The model under review builds one solid part; all positions refer to its coordinate system, in mm. A direction names the side the tool comes from. Coordinates: 2 decimals unless noted, no trailing zeros. Loops run counter-clockwise (first coordinate to the right, second up) from the corner with the lowest first, then second, coordinate; pieces in that order, holes last. Notation, with made-up numbers: M 75.25,-36 L 125.25,-36 A17 ccw 125.25,-17 Z; hole C -22.5,68.25 d10. An arc over 180 degrees is marked long. Use one line per item in the form item = value.
```python
from build123d import *

# Parameters (mm, degrees)
F1_DEPTH = 609.6
F2_R     = 5.08


with BuildPart() as f1:
    # F0 (on Front) → F1 (new body)
    with BuildSketch(Plane.XZ):
        Polygon((-76.2, -46.21704), (-76.2, -57.094753), (76.2, -57.094753), (76.2, -46.21704), (26.83735, -33.72637), (21.163462, -31.835258), (18.708812, -29.612178), (16.218112, -26.55388), (14.689744, -22.895062), (13.485576, -19.143616), (13.305501, -16.85449), (10.935693, -2.660843), (9.173225, 23.941404), (9.095304, 51.274587), (9.465817, 61.371074), (10.203332, 68.52603), (11.415046, 73.405639), (12.987001, 77.66302), (14.984693, 80.446691), (18.095852, 83.001115), (20.683027, 84.147327), (25.922873, 85.98128), (30.180251, 87.1275), (33.094916, 87.749728), (34.175634, 88.306465), (35.387348, 89.616426), (36.173157, 90.991981), (36.40228, 91.97448), (36.598587, 93.513711), (36.598872, 93.52041), (36.827176, 98.88458), (36.669851, 103.667696), (36.407496, 106.64783), (36.177806, 110.315693), (35.555092, 114.278253), (34.24468, 117.978737), (33.327476, 119.878062), (31.132972, 122.464971), (28.218115, 124.036569), (24.026078, 125.34602), (19.539378, 126.000454), (15.433662, 126.392808), (7.999516, 126.762047), (0, 126.762047), (-7.999516, 126.762047), (-15.433662, 126.392808), (-19.539378, 126.000454), (-24.026078, 125.34602), (-28.218115, 124.036569), (-31.132972, 122.464971), (-33.327476, 119.878062), (-34.24468, 117.978737), (-35.555092, 114.278253), (-36.177806, 110.315693), (-36.407496, 106.64783), (-36.669851, 103.667696), (-36.827176, 98.88458), (-36.598872, 93.52041), (-36.598587, 93.513711), (-36.40228, 91.97448), (-36.173157, 90.991981), (-35.387348, 89.616426), (-34.175634, 88.306465), (-33.094916, 87.749728), (-30.180251, 87.1275), (-25.922873, 85.98128), (-20.683027, 84.147327), (-18.095852, 83.001115), (-14.984693, 80.446691), (-12.987001, 77.66302), (-11.415046, 73.405639), (-10.203332, 68.52603), (-9.465817, 61.371074), (-9.095304, 51.274587), (-9.173225, 23.941404), (-10.935693, -2.660843), (-13.305501, -16.85449), (-13.485576, -19.143616), (-14.689744, -22.895062), (-16.218112, -26.55388), (-18.708812, -29.612178), (-21.163462, -31.835258), (-26.83735, -33.72637), align=None)
    extrude(amount=F1_DEPTH)

    # F2
    f2_edges = [f1.edges().sort_by_distance(p)[0] for p in [
        (76.2, -304.8, -46.21704),
        (-76.2, -304.8, -46.21704),
    ]]
    fillet(f2_edges, radius=F2_R)


solid = f1.part
```
1. Wall thickness on line 1 along X through (y, z) = (-460.5, 6.5); line 2 along Z through (x, y) = (-32, -50); line 3 along X through (y, z) = (-153, 96): over which ranges is each line inside the solid? List them lowest first. Write a range as from..to.
Response values:
line_1 = -10.33..10.33
line_2 = -57.09..-35.03, 87.52..121.44
line_3 = -36.7..36.7
2. Insertion check: P1, Ø4, axis at y = -84.5, z = 80.5, coming from the +X side; P2, Ø5, axis at y = -372.5, z = 104, coming from the -X side; P3, Ø12, axis at y = -184.5, z = 86.5, coming from the +X side. Each pin has a flat end and moves straight along its axis. Give the tip position at first contact, or say it passes through.
Response values:
P1 = 17.49
P2 = -36.74
P3 = 36.47
3. The part is to be moulded in two halves that separate along Z. For faces 4 (the face through (0, 0, 28)), 5 (the face through (-12.104, -300.533, -9.658)), 6 (the face through (12.137, -300.533, -9.857)), 7 (the face through (-1, -301, -57.095)), say which applies: pulls with the +Z half, pulls with the -Z half, needs draft (parallel to the pull), parting line crosses it, or undercut.
Response values:
face_4 = needs draft
face_5 = undercut
face_6 = undercut
face_7 = pulls with the -Z half
4. Add section B-B (x = 56). State the section outline as (y, z) points, then the cut area to 3 significant figures.
Response values:
outline = M -609.6,-57.09 L 0,-57.09 L 0,-41.11 L -609.6,-41.11 Z
area = 9,750 mm^2
5. Machinability: for faces 1 (the face through (-49.283, -300.533, -39.406)), 2 (the face through (49.92, -300.533, -39.567)), 3 (the face through (0, -301, 126.762)), which of the approach directions +Z, -Z, +X, -X, +Y, -Y give a long, thin tool a straight path to every point of the face, cutting with its end or side? Answer none if there is none.
Response values:
face_1 = -X, +Y, -Y
face_2 = +X, +Y, -Y
face_3 = +Z, +X, -X, +Y, -Y
6. Add section A-A (z = 9.5). State the section outline as (x, y) points.
Response values:
outline = M -10.13,-609.6 L 10.13,-609.6 L 10.13,0 L -10.13,0 Z
